```python
from build123d import *

# Parameters (mm, degrees)
F0_R      = 30.25
F1_DEPTH  = 3.5
F3_R      = 27.85
F3_R_2    = 25.35
F4_DEPTH  = 10
F5_DEPTH  = 6
F6_SIZE2  = 1.5
F6_SIZE   = 5
F8_DEPTH  = 10
F9_SIZE   = 0.99999
F10_DEPTH = 1.5
F11_SIZE  = 1


# Not quite as in the source:
# - a fillet or chamfer is up to 0.001 mm smaller than in the source, because OpenCascade refuses the exact size


with BuildPart() as f1:
    # F0 (on Top) → F1 (new body)
    with BuildSketch(Plane.XY):
        Circle(F0_R)
    extrude(amount=F1_DEPTH)

    # F3 (on face) → F4 (join)
    with BuildSketch(Plane.XY.offset(3.5)):
        Circle(F3_R)
        Circle(F3_R_2, mode=Mode.SUBTRACT)
    extrude(amount=F4_DEPTH)

    # F5 (add): a face of the model
    f5_faces = [f1.faces().sort_by_distance(p)[0] for p in [
        (-27.0622830458, 0, 13.5),
    ]]
    extrude(f5_faces, amount=F5_DEPTH)

    # F6
    f6_edges = [f1.edges().sort_by_distance(p)[0] for p in [
        (-27.85, 0, 19.5),
    ]]
    f6_side = f1.faces().sort_by_distance((-27.85, 0, 11.5))[0]
    chamfer(f6_edges, length=F6_SIZE, length2=F6_SIZE2, reference=f6_side)

    # F7 (on face) → F8 (join)
    with BuildSketch(Plane.XY.offset(3.5)):
        with BuildLine():
            ThreePointArc((27.85, 0), (27.8488778044, -0.250010074), (27.8455113079, -0.5))
            Line((27.8455113079, -0.5), (28.85, -0.5))
            Line((28.85, -0.5), (28.85, 0.5))
            Line((28.85, 0.5), (27.8455113079, 0.5))
            ThreePointArc((27.8455113079, 0.5), (27.8488778044, 0.250010074), (27.85, 0))
        make_face()
        with BuildLine():
            Line((-28.85, -0.5), (-27.8455113079, -0.5))
            ThreePointArc((-27.8455113079, -0.5), (-27.85, 0), (-27.8455113079, 0.5))
            Line((-27.8455113079, 0.5), (-28.85, 0.5))
            Line((-28.85, 0.5), (-28.85, -0.5))
        make_face()
        with BuildLine():
            Line((-0.5, -28.85), (0.5, -28.85))
            Line((0.5, -28.85), (0.5, -27.8455113079))
            ThreePointArc((0.5, -27.8455113079), (0, -27.85), (-0.5, -27.8455113079))
            Line((-0.5, -27.8455113079), (-0.5, -28.85))
        make_face()
        with BuildLine():
            ThreePointArc((-0.5, 27.8455113079), (0, 27.85), (0.5, 27.8455113079))
            Line((0.5, 27.8455113079), (0.5, 28.85))
            Line((0.5, 28.85), (-0.5, 28.85))
            Line((-0.5, 28.85), (-0.5, 27.8455113079))
        make_face()
    extrude(amount=F8_DEPTH)

    # F9 (size 1 in the source; OpenCascade refuses exactly that, so slightly less here)
    f9_edges = [f1.edges().sort_by_distance(p)[0] for p in [
        (28.85, 0, 13.5),
        (0, 28.85, 13.5),
        (-28.85, 0, 13.5),
        (0, -28.85, 13.5),
    ]]
    chamfer(f9_edges, length=F9_SIZE)

    # F10 (cut): a face of the model
    f10_faces = [f1.faces().sort_by_distance(p)[0] for p in [
        (0, 0, 3.5),
    ]]
    extrude(f10_faces, amount=-F10_DEPTH, mode=Mode.SUBTRACT)

    # F11
    f11_edges = [f1.edges().sort_by_distance(p)[0] for p in [
        (-30.25, 0, 0),
    ]]
    chamfer(f11_edges, length=F11_SIZE)


solid = f1.part
```
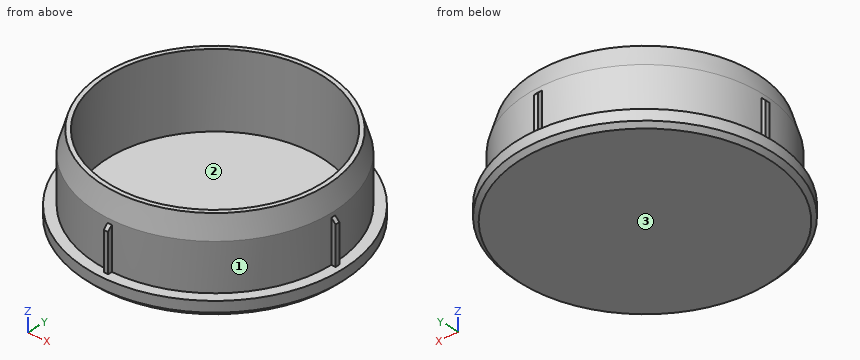
Geometry: final body of the model. Coordinates: model frame, mm. Face numbers are marked on the shaded views. Round coordinates to 2 decimals unless told otherwise and drop trailing zeros. Write each loop counter-clockwise with the first axis right and the second up, starting at its lowest first coordinate (ties: lowest second). Pieces come first, ordered by that corner, then holes. Notation, with made-up numbers: (11, 36.25) -> (62, 36.25) arc R20 ccw to (62, 69.25) -> close; hole circle Ø1 at (-39, 14). An arc over 180 degrees is marked (long way). Use CSV: the item, a comma, the result in double quotes. Start each with the question number.
Q1. Pull-direction query (Y, two-part tool) for the marked faces 1, 2 and 3; classes: pulls with the +Y half, pulls with the -Y half, needs draft (parallel to the pull), parting line crosses it, or undercut.
Q2. Section B-B (z = 17.5). Return loops of the section in (x, y).
Q3. First-contact query: pin 1 Ø1 at (x, z) = (21, 12) entering from -Y; pin 2 Ø5 at (x, z) = (8.5, 10) entering from +Y; pin 3 Ø1.5 at (x, y) = (-14, -19.5) entering from +Z. Flat tips, straight axial feed; report the tip coordinate or a pass-through.
Q4. Line query: L1, parallel to Y at x = 0, z = 10; L2, parallel to Z at x = -8, y = -21.5; L3, parallel to X at y = 17, z = 7.25. Output: solid intervals per line, ascending.
Q5. Section A-A (z = 4.5). Return loops of the section in (x, y), plus the area to 3 significant figures.
Result sheet:
1,face 1,"parting line crosses it"
1,face 2,"undercut"
1,face 3,"needs draft"
2,outline,"circle Ø53.9 at (0, 0); hole circle Ø50.7 at (0, 0)"
3,pin 1,"y = -18.85"
3,pin 2,"y = 27.2"
3,pin 3,"z = 2"
4,L1,"-28.85 to -25.35, 25.35 to 28.85"
4,L2,"0 to 2"
4,L3,"-22.06 to -18.8, 18.8 to 22.06"
5,outline,"(-28.85, -0.5) -> (-27.85, -0.5) arc R27.85 ccw to (-0.5, -27.85) -> (-0.5, -28.85) -> (0.5, -28.85) -> (0.5, -27.85) arc R27.85 ccw to (27.85, -0.5) -> (28.85, -0.5) -> (28.85, 0.5) -> (27.85, 0.5) arc R27.85 ccw to (0.5, 27.85) -> (0.5, 28.85) -> (-0.5, 28.85) -> (-0.5, 27.85) arc R27.85 ccw to (-27.85, 0.5) -> (-28.85, 0.5) -> close; hole circle Ø50.7 at (0, 0)"
5,area,"422 mm²"
